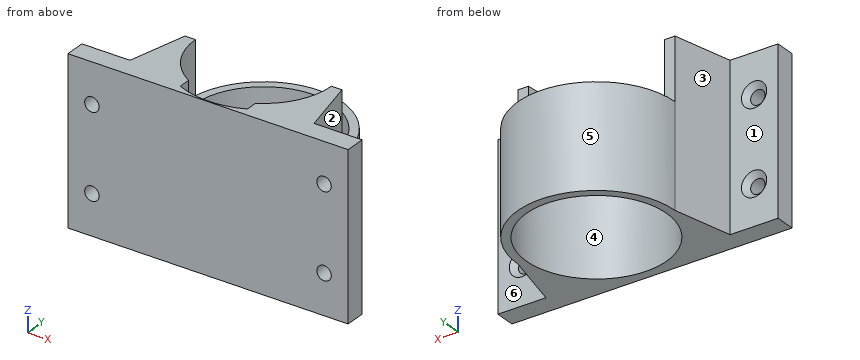
from build123d import *

# Parameters (mm, degrees)
SKETCH1_R                                       = 17.5
BOSS_EXTRUDE9_DEPTH                             = 25.5
BOSS_EXTRUDE10_DEPTH                            = 15.4
BOSS_EXTRUDE10_DEPTH_BACK                       = 25.5
CSK_FOR_M3_FLAT_HEAD_MACHINE_SCREW1_D           = 3.6
CSK_FOR_M3_FLAT_HEAD_MACHINE_SCREW1_CSINK_D     = 6.3
CSK_FOR_M3_FLAT_HEAD_MACHINE_SCREW1_CSINK_ANGLE = 90
CSK_FOR_M3_FLAT_HEAD_MACHINE_SCREW2_D           = 3.6
CSK_FOR_M3_FLAT_HEAD_MACHINE_SCREW2_CSINK_D     = 6.3
CSK_FOR_M3_FLAT_HEAD_MACHINE_SCREW2_CSINK_ANGLE = 90
BOSS_EXTRUDE12_DEPTH                            = 15.4


with BuildPart() as part:
    # Sketch1 → Boss-Extrude9 (new body)
    with BuildSketch(Plane.XY):
        with BuildLine():
            ThreePointArc((-19.6, 19.8), (0, 39.4), (19.6, 19.8))
            ThreePointArc((19.6, 19.8), (0, 0.2), (-19.6, 19.8))
        make_face()
        with Locations((0, 19.8)):
            Circle(SKETCH1_R, mode=Mode.SUBTRACT)
    extrude(amount=-BOSS_EXTRUDE9_DEPTH)

    # Sketch1_15 → Boss-Extrude10 (add, two sides: drawn at the far end of the back side and taken through both)
    with BuildSketch(Plane.XY.offset(-BOSS_EXTRUDE10_DEPTH_BACK)):
        with BuildLine():
            Line((-23, 5), (-35, 5))
            Line((-35, 5), (-35, 0))
            Line((-35, 0), (35, 0))
            Line((35, 0), (35, 5))
            Line((35, 5), (23, 5))
            Line((23, 5), (19.6, 19.8))
            ThreePointArc((19.6, 19.8), (0, 0.2), (-19.6, 19.8))
            Line((-19.6, 19.8), (-23, 5))
        make_face()
    extrude(amount=BOSS_EXTRUDE10_DEPTH + BOSS_EXTRUDE10_DEPTH_BACK)

    # CSK for M3 Flat Head Machine Screw1 (through all)
    with Locations(Plane(origin=(0, 5, 0), x_dir=(1, 0, 0), z_dir=(0, 1, 0))):
        with Locations((-29, 15.5), (-29, -5.4)):
            CounterSinkHole(CSK_FOR_M3_FLAT_HEAD_MACHINE_SCREW1_D / 2, CSK_FOR_M3_FLAT_HEAD_MACHINE_SCREW1_CSINK_D / 2, counter_sink_angle=CSK_FOR_M3_FLAT_HEAD_MACHINE_SCREW1_CSINK_ANGLE)

    # CSK for M3 Flat Head Machine Screw2 (through all)
    with Locations(Plane(origin=(0, 5, 0), x_dir=(1, 0, 0), z_dir=(0, 1, 0))):
        with Locations((29, -5.4), (29, 15.5)):
            CounterSinkHole(CSK_FOR_M3_FLAT_HEAD_MACHINE_SCREW2_D / 2, CSK_FOR_M3_FLAT_HEAD_MACHINE_SCREW2_CSINK_D / 2, counter_sink_angle=CSK_FOR_M3_FLAT_HEAD_MACHINE_SCREW2_CSINK_ANGLE)

    # Sketch20 → Boss-Extrude12 (add)
    with BuildSketch(Plane.XY):
        with BuildLine():
            ThreePointArc((17, 19.8), (14.683180189, 11.232373751), (8.364209467, 5))
            Line((8.364209467, 5), (8.364209467, 2.074312425))
            ThreePointArc((8.364209467, 2.074312425), (16.554433025, 9.30663318), (19.6, 19.8))
            Line((19.6, 19.8), (17, 19.8))
        make_face()
        with BuildLine():
            Line((-8.364209467, 2.074312425), (-8.364209467, 5))
            ThreePointArc((-8.364209467, 5), (-14.683180189, 11.232373751), (-17, 19.8))
            Line((-17, 19.8), (-19.6, 19.8))
            ThreePointArc((-19.6, 19.8), (-16.554433025, 9.30663318), (-8.364209467, 2.074312425))
        make_face()
    extrude(amount=BOSS_EXTRUDE12_DEPTH)


solid = part.part
Read the model definition and answer for the solid it produces. Units are mm, in the model's axes. Face numbers are marked on the shaded views. A direction names the side the tool comes from. Round coordinates to 2 decimals unless told otherwise and drop trailing zeros. Loops run counter-clockwise (first coordinate to the right, second up) from the corner with the lowest first, then second, coordinate; pieces in that order, holes last. Notation, with made-up numbers: (52.5, 6.25) - (79.5, 6.25) arc R14 cw to (79.5, 25.25) - close; hole circle Ø8 at (27.25, 85). An arc over 180 degrees is marked (long way). One line per question, with ' | ' between items. Start each with the question number.
Q1. Section C-C on z = 5.4 is taken. Give the vertices of the cut face in (x, y), plus the area to 3 significant figures.
Q2. Section D-D on z = -6.5 is taken. Give the vertices of the cut face in (x, y), plus the area to 3 significant figures.
Q3. For the marked faces 1 and 2, determine the directions among +Z, -Z, +X, -X, +Y, -Y from which every point of the face is accessible in a straight line to the end or side of a thin tool.
Q4. Section B-B on z = -15.5 is taken. Give the vertices of the cut face in (x, y), plus the area to 3 significant figures.
Q5. Flat-ended cylindrical pins translate along their axes: pin 1 (10 mm diameter, centred on x = -5.5, z = 10.5, fed in from +Y); pin 2 (1.3 mm diameter, centred on x = 18, z = 9, fed in from +Y); pin 3 (2 mm diameter, centred on y = 35, z = -13, fed in from +X); pin 4 (2 mm diameter, centred on y = 25.5, z = 2.5, fed in from -X). Find the tip coordinate at first contact, or state that the pin passes through.
Q6. For a pull along X with two mould halves and no side action, classify the marked faces 3, 4, 5 and 6 as +X half, -X half, draft (parallel to the pull), parting line (faces both ways), or undercut.
Q7. Find the intervals of material crossed by L1, parallel to Z at x = 29, y = 1; L2, parallel to X at y = 2.1, z = 5.4; L3, parallel to X at y = 2.1, z = -15.5, in increasing order.
Q8. Section A-A on x = 29 is taken. Give the vertices of the cut face in (y, z), plus the area to 3 significant figures.
Established:
1) outline: (-35, 0) - (-30.8, 0) - (-30.8, 3.65) - (-32.15, 5) - (-35, 5) - close; (-27.2, 0) - (27.2, 0) - (27.2, 3.65) - (25.85, 5) - (23, 5) - (19.6, 19.8) - (17, 19.8) arc R17 cw to (8.36, 5) - (8.36, 2.07) arc R19.6 cw to (-8.36, 2.07) - (-8.36, 5) arc R17 cw to (-17, 19.8) - (-19.6, 19.8) - (-23, 5) - (-25.85, 5) - (-27.2, 3.65) - close; (30.8, 0) - (35, 0) - (35, 5) - (32.15, 5) - (30.8, 3.65) - close | area: 442 mm²
2) outline: (-35, 0) - (35, 0) - (35, 5) - (23, 5) - (19.6, 19.8) arc R19.6 ccw to (-19.6, 19.8) - (-23, 5) - (-35, 5) - close; hole circle Ø35 at (0, 19.8) | area: 622 mm²
3) face 1: +Z, -Z, -X, +Y | face 2: +Z, -Z, +X, +Y
4) outline: (-35, 0) - (-30.8, 0) - (-30.8, 3.65) - (-32.15, 5) - (-35, 5) - close; (-27.2, 0) - (27.2, 0) - (27.2, 3.65) - (25.85, 5) - (23, 5) - (19.6, 19.8) arc R19.6 ccw to (-19.6, 19.8) - (-23, 5) - (-25.85, 5) - (-27.2, 3.65) - close; (30.8, 0) - (35, 0) - (35, 5) - (32.15, 5) - (30.8, 3.65) - close; hole circle Ø35 at (0, 19.8) | area: 582 mm²
5) pin 1: y = 6.43 | pin 2: y = 19.8 | pin 3: x = 13.51 | pin 4: through
6) face 3: -X half | face 4: undercut | face 5: parting line | face 6: draft
7) L1: -25.5 to -17.3, -13.7 to 3.6, 7.2 to 15.4 | L2: -35 to -30.8, -27.2 to -8.36, 8.36 to 27.2, 30.8 to 35 | L3: -35 to -30.8, -27.2 to 27.2, 30.8 to 35
8) outline: (0, -25.5) - (5, -25.5) - (5, -18.65) - (3.65, -17.3) - (0, -17.3) - close; (0, -13.7) - (3.65, -13.7) - (5, -12.35) - (5, 2.25) - (3.65, 3.6) - (0, 3.6) - close; (0, 7.2) - (3.65, 7.2) - (5, 8.55) - (5, 15.4) - (0, 15.4) - close | area: 165 mm²
